Build history of the part. All positions in model axes, mm. Face numbers are marked on the shaded views. Give positions to 0.01 mm unless a question says otherwise; leave off trailing zeros. Loops run counter-clockwise (first coordinate to the right, second up) from the corner with the lowest first, then second, coordinate; pieces in that order, holes last. Notation, with made-up numbers: (13.5, 7) -> (55.5, 7) arc R17 ccw to (55.5, 26) -> close; hole circle Ø7 at (58.5, 62.25). An arc over 180 degrees is marked (long way). Answer in a Markdown table with one row per item. Add a question column.
from build123d import *

# Parameters (mm, degrees)
F0_W     = 45.0391359627
F0_H     = 63.62747401
F1_DEPTH = 170.4394621775
F3_D     = 25
F3_DEPTH = 50
F3_TIP   = 7.5107577378
F5_D     = 20


with BuildPart() as f1:
    # F0 (on Right) → F1 (new body, symmetric)
    with BuildSketch(Plane.YZ):
        Rectangle(F0_W, F0_H)
    extrude(amount=F1_DEPTH, both=True)

    # F3
    with Locations(Plane.YZ.offset(170.4394621775)):
        with Locations((0, 0)):
            Hole(F3_D / 2, depth=F3_DEPTH)
            with Locations((0, 0, -(F3_DEPTH + F3_TIP / 2))):  # 118° drill point
                Cone(0, F3_D / 2, F3_TIP, mode=Mode.SUBTRACT)

    # F5 (through all)
    with Locations(Plane.YZ.offset(170.4394621775)):
        with Locations((0.0467002392, 0.2690460533)):
            Hole(F5_D / 2)


solid = f1.part
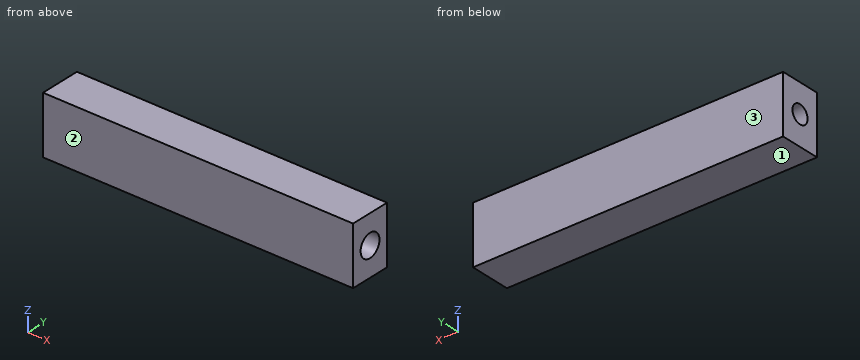
(1) Two-plate mould, pull along Y, no slides. Class the marked faces 1, 2 and 3: released by +Y, released by -Y, zero draft, split by the parting line, or undercut.
(2) Saw through at C-C, the plane x = 52.5. List the corners of the cut face in (y, z), then the cut area to 3 significant figures.
(3) Saw through at B-B, the plane x = 139. List the corners of the cut face in (y, z), then the cut area to 3 significant figures.
(4) Wall check: line 1 along Z through (x, y) = (140, 0); line 2 along Y through (x, z) = (154, 0); line 3 along Z through (x, y) = (37, -8). Give the ranges that are in metal, low to high. Write a range as from..to.
(5) Saw through at A-A, the plane y = 0. List the corners of the cut face in (x, z).
Worked answers:
| question | item | result |
|---|---|---|
| 1 | face 1 | zero draft |
| 1 | face 2 | released by -Y |
| 1 | face 3 | released by +Y |
| 2 | outline | (-22.52, -31.81) -> (22.52, -31.81) -> (22.52, 31.81) -> (-22.52, 31.81) -> close; hole circle Ø20 at (0.05, 0.27) |
| 2 | area | 2,550 mm^2 |
| 3 | outline | (-22.52, -31.81) -> (22.52, -31.81) -> (22.52, 31.81) -> (-22.52, 31.81) -> close; hole circle Ø25 at (0, 0) |
| 3 | area | 2,370 mm^2 |
| 4 | line 1 | -31.81..-12.5, 12.5..31.81 |
| 4 | line 2 | -22.52..-12.5, 12.5..22.52 |
| 4 | line 3 | -31.81..-5.67, 6.21..31.81 |
| 5 | outline | (-170.44, -31.81) -> (170.44, -31.81) -> (170.44, -12.5) -> (120.44, -12.5) -> (118.78, -9.73) -> (-170.44, -9.73) -> close; (-170.44, 10.27) -> (119.1, 10.27) -> (120.44, 12.5) -> (170.44, 12.5) -> (170.44, 31.81) -> (-170.44, 31.81) -> close |
